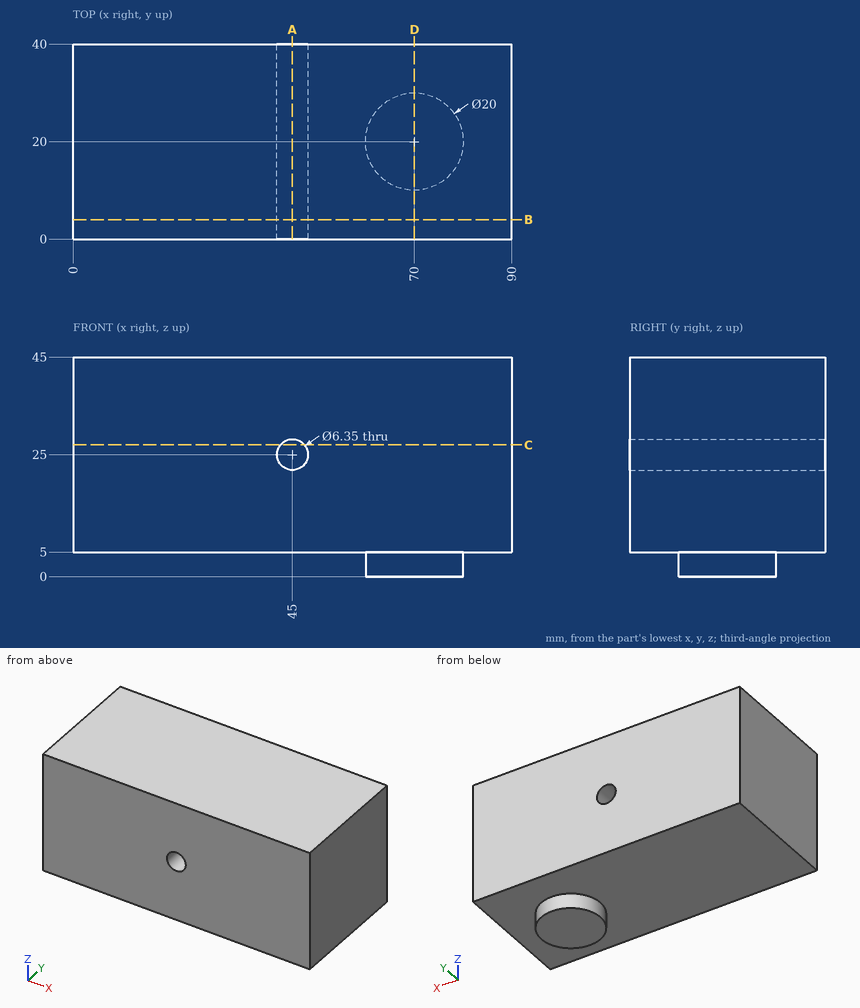
Input: dimensioned drawing with shaded views. Units: mm. Origin: part minimum x, y, z. Round coordinates to 2 decimals unless told otherwise and drop trailing zeros. Order: outer loops, then holes, each group sorted by start corner. A loop starts at its lowest first (then second) coordinate and runs counter-clockwise, first axis right, second up. Notation, with made-up numbers: (-32.5, 17) -> (-28.5, 17) arc R26 cw to (-28.5, 47) -> close; hole circle Ø2 at (41.25, 66.5). An arc over 180 degrees is marked (long way). Put each result on its own line as item: value. Start each with the question number.
Q1. Section C-C on z = 27. Return the cut outline in (x, y), and give its area (3 significant figures).
Q2. Section D-D on x = 70. Return the cut outline in (y, z), and give its area (3 significant figures).
Q3. Section A-A on x = 45. Return the cut outline in (y, z) (3 decimals), and give its area (3 significant figures).
Q4. Section B-B on y = 4. Return the cut outline in (x, z) (3 decimals).
Q5. First-contact query: pin 1 (4 mm diameter, centred on x = 71, y = 25, fed in from -Z); pin 2 (1.5 mm diameter, centred on x = 11.5, y = 29.5, fed in from -Z). Flat tips, straight axial feed; report the tip coordinate or a pass-through.
Q6. Line query: probe 1 along X at (y, z) = (10, 25) (3 decimals); probe 2 along Z at (x, y) = (45, 34) (3 decimals); probe 3 along Z at (x, y) = (61.5, 2). Output: solid intervals per line, ascending.
Ans:
1. outline: (0, 0) -> (42.53, 0) -> (42.53, 40) -> (0, 40) -> close; (47.47, 0) -> (90, 0) -> (90, 40) -> (47.47, 40) -> close
1. area: 3,400 mm2
2. outline: (0, 5) -> (10, 5) -> (10, 0) -> (30, 0) -> (30, 5) -> (40, 5) -> (40, 45) -> (0, 45) -> close
2. area: 1,700 mm2
3. outline: (0, 5) -> (40, 5) -> (40, 21.825) -> (0, 21.825) -> close; (0, 28.175) -> (40, 28.175) -> (40, 45) -> (0, 45) -> close
3. area: 1,350 mm2
4. outline: (0, 5) -> (90, 5) -> (90, 45) -> (0, 45) -> close; hole circle Ø6.35 at (45, 25)
5. pin 1: stops at z = 0
5. pin 2: stops at z = 5
6. probe 1: x = 0 to 41.825, 48.175 to 90
6. probe 2: z = 5 to 21.825, 28.175 to 45
6. probe 3: z = 5 to 45
